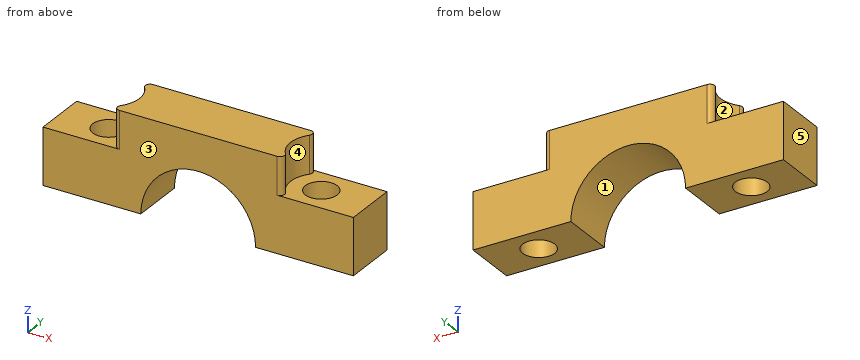
```python
from build123d import *

# Parameters (mm, degrees)
BOSS_EXTRUDE1_DEPTH  = 5.8
M3_CLEARANCE_HOLE1_D = 3.4
CUT_EXTRUDE1_DEPTH   = 4
FILLET1_R            = 0.5


with BuildPart() as part:
    # Sketch1 → Boss-Extrude1 (new body)
    with BuildSketch(Plane(origin=(0, 0, 0), x_dir=(1, 0, 0), z_dir=(0, 1, 0))):
        with BuildLine():
            Line((-16.5, 0), (16.5, 0))
            Line((16.5, 0), (16.5, 10))
            Line((16.5, 10), (6.1, 10))
            ThreePointArc((6.1, 10), (0, 3.9), (-6.1, 10))
            Line((-6.1, 10), (-16.5, 10))
            Line((-16.5, 10), (-16.5, 0))
        make_face()
    extrude(amount=BOSS_EXTRUDE1_DEPTH)

    # M3 Clearance Hole1 (through all)
    with Locations(Plane.XY):
        with Locations((-11.3, 2.9), (11.3, 2.9)):
            Hole(M3_CLEARANCE_HOLE1_D / 2)

    # Sketch5 → Cut-Extrude1 (cut)
    with BuildSketch(Plane.XY):
        with BuildLine():
            Line((-9.778282221, 5.8), (-16.5, 5.8))
            Line((-16.5, 5.8), (-16.5, 0))
            Line((-16.5, 0), (-9.778282221, 0))
            ThreePointArc((-9.778282221, 0), (-8.025, 2.9), (-9.778282221, 5.8))
        make_face()
        with BuildLine():
            Line((16.5, 0), (9.778282221, 0))
            ThreePointArc((9.778282221, 0), (8.025, 2.9), (9.778282221, 5.8))
            Line((9.778282221, 5.8), (16.5, 5.8))
            Line((16.5, 5.8), (16.5, 0))
        make_face()
    extrude(amount=-CUT_EXTRUDE1_DEPTH, mode=Mode.SUBTRACT)

    # Fillet1
    fillet1_edges = [part.edges().sort_by_distance(p)[0] for p in [
        (-9.778282221, 5.8, -2),
        (-9.778282221, 0, -2),
        (9.778282221, 0, -2),
        (9.778282221, 5.8, -2),
    ]]
    fillet(fillet1_edges, radius=FILLET1_R)


solid = part.part
```
Geometry check sheet. Reference: the model listing, model coordinates, mm. Face numbers are marked on the shaded views. A direction names the side the tool comes from. Coordinates: 2 decimals unless noted, no trailing zeros. Loops run counter-clockwise (first coordinate to the right, second up) from the corner with the lowest first, then second, coordinate; pieces in that order, holes last. Notation, with made-up numbers: (58.5, 30) - (116.5, 30) arc R14 cw to (116.5, 34) - close; hole circle Ø10 at (27, -30.5). An arc over 180 degrees is marked (long way). One line per item, written item: value. Start each with the question number.
(1) Cross-section at A-A on z = -5.75. Enter the section's corners in (x, y), plus the area to 3 significant figures.
(2) Tool access check on the marked faces 4 and 5. Record the directions out of +Z, -Z, +X, -X, +Y, -Y that give a thin tool (end or side, any length) a straight path to the whole face; none if there is none.
(3) Cross-section at C-C on x = 11.3. Enter the section's corners in (y, z).
(4) Material ranges on line 1 (Y direction, x = -11.3, z = -5.6); line 2 (X direction, y = 3.05, z = -8.75); line 3 (X direction, y = 4.2, z = -9.25), recorded low to high. Write a range as [from, to].
(5) Cross-section at B-B on y = 2.9. Enter the section's corners in (x, z) (3 decimals).
(6) Mould release check, pull along Y, two halves, no side actions. Record for the marked faces 1, 2 and 3: released by +Y, released by -Y, zero draft, split by the parting line, or undercut.
(7) Cross-section at D-D on z = -1. Enter the section's corners in (x, y) (3 decimals), plus the area to 3 significant figures.
(8) Depth check by flat-ended pin: P1, Ø3, axis at x = 12, y = 3.5, coming from the +Z side; P2, Ø1.5, axis at y = 3.5, z = -2.5, coming from the +X side. Enter the tip coordinate at first touch or a pass-through.
Results below:
1. outline: (-16.5, 0) - (-4.38, 0) - (-4.38, 5.8) - (-16.5, 5.8) - close; (4.38, 0) - (16.5, 0) - (16.5, 5.8) - (4.38, 5.8) - close; hole circle Ø3.4 at (-11.3, 2.9); hole circle Ø3.4 at (11.3, 2.9)
1. area: 122 mm2
2. face 4: +Z, +X
2. face 5: +Z, -Z, -X, +Y, -Y
3. outline: (0, -10) - (1.2, -10) - (1.2, -4) - (0, -4) - close; (4.6, -10) - (5.8, -10) - (5.8, -4) - (4.6, -4) - close
4. line 1: y = [0, 1.2], [4.6, 5.8]
4. line 2: x = [-16.5, -12.99], [-9.61, -5.97], [5.97, 9.61], [12.99, 16.5]
4. line 3: x = [-16.5, -12.4], [-10.2, -6.05], [6.05, 10.2], [12.4, 16.5]
5. outline: (-16.5, -10) - (-13, -10) - (-13, -4) - (-16.5, -4) - close; (-9.6, -10) - (-6.1, -10) arc R6.1 cw to (6.1, -10) - (9.6, -10) - (9.6, -4) - (8.025, -4) - (8.025, 0) - (-8.025, 0) - (-8.025, -4) - (-9.6, -4) - close; (13, -10) - (16.5, -10) - (16.5, -4) - (13, -4) - close
6. face 1: zero draft
6. face 2: undercut
6. face 3: released by -Y
7. outline: (-8.772, 0.818) arc R0.5 ccw to (-8.386, 0) - (8.386, 0) arc R0.5 ccw to (8.772, 0.818) arc R3.275 cw to (8.772, 4.982) arc R0.5 ccw to (8.386, 5.8) - (-8.386, 5.8) arc R0.5 ccw to (-8.772, 4.982) arc R3.275 cw to start
7. area: 97.6 mm2
8. P1: stops at z = -4
8. P2: stops at x = 8.32
